Input: part model. Units: mm. Frame: model coordinates. Give positions to 0.01 mm unless a question says otherwise; leave off trailing zeros. Loops run counter-clockwise (first coordinate to the right, second up) from the corner with the lowest first, then second, coordinate; pieces in that order, holes last. Notation, with made-up numbers: M -35.5,-5 L -2.5,-5 A30 cw -2.5,30 Z; hole C -10,-13 d6. An arc over 180 degrees is marked long. Use a Markdown table: item, result. Add a question column.
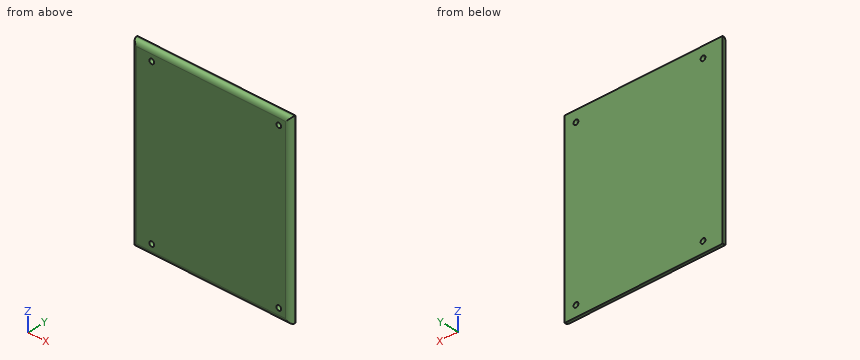
from build123d import *

# Parameters (mm, degrees)
F0_W     = 70
F0_H     = 80
F0_R     = 1.05
F1_DEPTH = 2.5
F2_R     = 2


with BuildPart() as f1:
    # F0 (on Front) → F1 (new body)
    with BuildSketch(Plane.XZ):
        with Locations((-6.523669, 13.454498)):
            Rectangle(F0_W, F0_H)
        with Locations((-32.844519, -21.745502)):
            Circle(F0_R, mode=Mode.SUBTRACT)
        with Locations((23.476331, -21.745502)):
            Circle(F0_R, mode=Mode.SUBTRACT)
        with Locations((-32.844519, 48.654498)):
            Circle(F0_R, mode=Mode.SUBTRACT)
        with Locations((23.476331, 48.654498)):
            Circle(F0_R, mode=Mode.SUBTRACT)
    extrude(amount=F1_DEPTH)

    # F2
    f2_edges = [f1.edges().sort_by_distance(p)[0] for p in [
        (-6.523669, -2.5, 53.454498),
        (-41.523669, -2.5, 13.454498),
        (-6.523669, -2.5, -26.545502),
        (28.476331, -2.5, 13.454498),
    ]]
    fillet(f2_edges, radius=F2_R)


solid = f1.part
1) Ray query, line 1 (X direction, y = -1.1, z = 49.5); line 2 (X direction, y = -2.05, z = -21); line 3 (Z direction, x = 24, y = -0.35). Return the intervals inside material, ascending. Write a range as [from, to].
2) Section query A-A, the plane x = 23.5. Return the cut outline in (y, z), and give its area (3 significant figures).
3) Section query B-B, the plane y = -1.95. Return the cut outline in (x, z).
Entries:
| question | item | result |
|---|---|---|
| 1 | line 1 | x = [-41.43, -33.47], [-32.22, 22.85], [24.1, 28.38] |
| 1 | line 2 | x = [-40.79, -33.58], [-32.11, 22.74], [24.22, 27.74] |
| 1 | line 3 | z = [-26.55, -22.66], [-20.84, 47.74], [49.56, 53.45] |
| 2 | outline | M -2.5,-24.55 A2 ccw -0.5,-26.55 L 0,-26.55 L 0,-22.8 L -2.5,-22.8 Z; M -2.5,-20.7 L 0,-20.7 L 0,47.6 L -2.5,47.6 Z; M -2.5,49.7 L 0,49.7 L 0,53.45 L -0.5,53.45 A2 ccw -2.5,51.45 Z |
| 2 | area | 188 mm² |
| 3 | outline | M -40.9,-25.92 L 27.85,-25.92 L 27.85,52.83 L -40.9,52.83 Z; hole C -32.84,-21.75 d2.1; hole C -32.84,48.65 d2.1; hole C 23.48,-21.75 d2.1; hole C 23.48,48.65 d2.1 |
